Part model, mm, in its own coordinate system. A direction names the side the tool comes from. Coordinates: 2 decimals unless noted, no trailing zeros. Loops run counter-clockwise (first coordinate to the right, second up) from the corner with the lowest first, then second, coordinate; pieces in that order, holes last. Notation, with made-up numbers: M -12.5,12 L 34.5,12 A24 ccw 34.5,50 Z; hole C 4,-23.5 d6. An arc over 180 degrees is marked long. Use a Markdown table: item, result. Add a question column.
1) Pull direction Y, two halves, no side cores. Call faces 5 (the flat face through (-1.94, 5.35, 14.79)), 6 (the flat face through (0, -3, 0)), 7 (the cylindrical face through (-5.284, 3.551, 14.79)), 8 (the cylindrical face through (1.225, -6.247, 14.79)): released by +Y, released by -Y, zero draft, split by the parting line, or undercut.
2) Tool access for faces 1 (the cylindrical face through (1, 4.9, 14.8)), 2 (the flat face through (0.22, -5.67, 14.79)), 3 (the flat face through (-5.67, -0.22, 14.79)), 4 (the flat face through (5.153, -2.409, 14.79)): list every direction of +Z, -Z, +X, -X, +Y, -Y with a clear straight run to the whole face (end or side of a thin tool).
3) Wall check: probe 1 along Y at (x, z) = (-1.75, 23); probe 2 along Y at (x, z) = (-4, 24.25) (3 decimals); probe 3 along Y at (x, z) = (-3.5, 17.5). Give the ranges that are in metal, low to high. Write a range as from..to.
4) Band-saw the part on C-C (y = 1). List the corners of the cut face in (x, z), plus the area to 3 significant figures.
5) Pin check, flat tips, straight feed: pin 1 Ø2 at (x, z) = (3, 11.5) entering from +Y; pin 2 Ø5 at (x, z) = (-3.5, 24) entering from +Y; pin 3 Ø4 at (x, y) = (-1.5, -1) entering from -Z; pin 4 Ø6 at (x, z) = (-4.5, 20.5) entering from +Y. Stop position of each tip, or through.
6) Band-saw the part on A-A (x = 1.25). List the corners of the cut face in (y, z), plus the area to 3 significant figures.
Solid Edge part; units mm, degrees
sketch "Sketch1" plane through (0, 0, 0) normal (0, 0, 1) x (1, 0, 0)
  line L0 (5, 0) -> (6.3507, 0.4441)
  arc A0 (6.0546, 1.9673) -> (6.3507, 0.4441) centre (0, 0) cw
  line L1 (6.0546, 1.9673) -> (4.6194, 1.9134)
  arc A1 (3.5355, 3.5355) -> (4.6194, 1.9134) centre (0, 0) cw
  line L2 (3.5355, 3.5355) -> (4.1766, 4.8046)
  arc A2 (2.8902, 5.6723) -> (4.1766, 4.8046) centre (0, 0) cw
  line L3 (2.8902, 5.6723) -> (1.9134, 4.6194)
  arc A3 (0, 5) -> (1.9134, 4.6194) centre (0, 0) cw
  line L4 (0, 5) -> (-0.4441, 6.3507)
  arc A4 (-1.9673, 6.0546) -> (-0.4441, 6.3507) centre (0, 0) cw
  line L5 (-1.9673, 6.0546) -> (-1.9134, 4.6194)
  arc A5 (-3.5355, 3.5355) -> (-1.9134, 4.6194) centre (0, 0) cw
  line L6 (-3.5355, 3.5355) -> (-4.8046, 4.1766)
  arc A6 (-5.6723, 2.8902) -> (-4.8046, 4.1766) centre (0, 0) cw
  line L7 (-5.6723, 2.8902) -> (-4.6194, 1.9134)
  arc A7 (-5, 0) -> (-4.6194, 1.9134) centre (0, 0) cw
  line L8 (-5, 0) -> (-6.3507, -0.4441)
  arc A8 (-6.0546, -1.9673) -> (-6.3507, -0.4441) centre (0, 0) cw
  line L9 (-6.0546, -1.9673) -> (-4.6194, -1.9134)
  arc A9 (-3.5355, -3.5355) -> (-4.6194, -1.9134) centre (0, 0) cw
  line L10 (-3.5355, -3.5355) -> (-4.1766, -4.8046)
  arc A10 (-2.8902, -5.6723) -> (-4.1766, -4.8046) centre (0, 0) cw
  line L11 (-2.8902, -5.6723) -> (-1.9134, -4.6194)
  arc A11 (0, -5) -> (-1.9134, -4.6194) centre (0, 0) cw
  line L12 (0, -5) -> (0.4441, -6.3507)
  arc A12 (1.9673, -6.0546) -> (0.4441, -6.3507) centre (0, 0) cw
  line L13 (1.9673, -6.0546) -> (1.9134, -4.6194)
  arc A13 (3.5355, -3.5355) -> (1.9134, -4.6194) centre (0, 0) cw
  line L14 (3.5355, -3.5355) -> (4.8046, -4.1766)
  arc A14 (5.6723, -2.8902) -> (4.8046, -4.1766) centre (0, 0) cw
  line L15 (5.6723, -2.8902) -> (4.6194, -1.9134)
  arc A15 (5, 0) -> (4.6194, -1.9134) centre (0, 0) cw
extrude "Protrusion1" add sketch "Sketch1" along normal blind 30
sketch "Sketch2" plane through (0, 0, 30) normal (0, 0, 1) x (1, 0, 0)
  circle A0 centre (0, 0) radius 2.5
extrude "Cutout1" cut sketch "Sketch2" against normal through all
Entries:
| question | item | result |
|---|---|---|
| 1 | face 5 | undercut |
| 1 | face 6 | zero draft |
| 1 | face 7 | released by +Y |
| 1 | face 8 | released by -Y |
| 2 | face 1 | +Z, -Z, +Y |
| 2 | face 2 | +Z, -Z, -Y |
| 2 | face 3 | +Z, -Z, -X |
| 2 | face 4 | +Z, -Z, +X |
| 3 | probe 1 | -4.68..-1.79, 1.79..6.12 |
| 3 | probe 2 | -4.953..-4.455, -3..3.77 |
| 3 | probe 3 | -5.32..3.57 |
| 4 | outline | M -4.9,0 L -2.29,0 L -2.29,30 L -4.9,30 Z; M 2.29,0 L 6.29,0 L 6.29,30 L 2.29,30 Z |
| 4 | area | 198 mm2 |
| 5 | pin 1 | y = 5.67 |
| 5 | pin 2 | y = 6.29 |
| 5 | pin 3 | z = 0 |
| 5 | pin 4 | y = 6.19 |
| 6 | outline | M -6.24,0 L -2.17,0 L -2.17,30 L -6.24,30 Z; M 2.17,0 L 4.84,0 L 4.84,30 L 2.17,30 Z |
| 6 | area | 203 mm2 |
